The listing builds one solid part. Answer for the finished solid, in the listing's coordinates (mm). Round coordinates to 2 decimals unless told otherwise and drop trailing zeros. Answer in a Markdown table with one row per item. Add a question column.
```python
from build123d import *

# Parameters (mm, degrees)
F1_DEPTH = 3.175
F2_D     = 7.1374
F3_R     = 5.08
F4_D     = 5.6134


# Not quite as in the source:
# - a feature names something its author has since deleted; it is built from what else it names


with BuildPart() as f1:
    # F0 (on Top) → F1 (new body)
    with BuildSketch(Plane.XY):
        Polygon((0, 1181.1), (0, 38.1), (800.1, 38.1), (800.1, 1181.1), (749.3, 1181.1), (749.3, 1155.7), (50.8, 1155.7), (50.8, 1181.1), align=None)
    extrude(amount=F1_DEPTH)

    # F2 (through all)
    with Locations(Plane(origin=(0, 0, 0), x_dir=(1, 0, 0), z_dir=(0, 0, -1))):
        with Locations((25.4, -1168.4), (92.075, -965.2), (117.475, -965.2), (276.225, -965.2), (301.625, -965.2), (460.375, -965.2), (485.775, -965.2), (644.525, -965.2), (669.925, -965.2), (774.7, -1168.4), (669.925, -660.4), (644.525, -660.4), (485.775, -660.4), (460.375, -660.4), (301.625, -660.4), (276.225, -660.4), (117.475, -660.4), (92.075, -660.4), (92.075, -355.6), (117.475, -355.6), (276.225, -355.6), (301.625, -355.6), (460.375, -355.6), (485.775, -355.6), (644.525, -355.6), (669.925, -355.6), (669.925, -50.8), (644.525, -50.8), (485.775, -50.8), (460.375, -50.8), (301.625, -50.8), (276.225, -50.8), (117.475, -50.8), (92.075, -50.8), (774.7, -1079.5), (774.7, -1054.1), (774.7, -774.7), (774.7, -749.3), (774.7, -469.9), (774.7, -444.5), (774.7, -165.1), (774.7, -139.7), (180.975, -965.2), (28.575, -965.2), (212.725, -965.2), (104.775, -1108.075), (288.925, -1108.075), (365.125, -965.2), (396.875, -965.2), (473.075, -1108.075), (549.275, -965.2), (581.025, -965.2), (657.225, -1108.075), (733.425, -965.2), (657.225, -803.275), (473.075, -803.275), (288.925, -803.275), (104.775, -803.275), (28.575, -660.4), (180.975, -660.4), (212.725, -660.4), (365.125, -660.4), (396.875, -660.4), (549.275, -660.4), (581.025, -660.4), (733.425, -660.4), (657.225, -498.475), (473.075, -498.475), (288.925, -498.475), (104.775, -498.475), (28.575, -355.6), (180.975, -355.6), (212.725, -355.6), (365.125, -355.6), (396.875, -355.6), (549.275, -355.6), (581.025, -355.6), (733.425, -355.6), (104.775, -193.675), (288.925, -193.675), (473.075, -193.675), (657.225, -193.675), (733.425, -50.8), (581.025, -50.8), (549.275, -50.8), (396.875, -50.8), (365.125, -50.8), (212.725, -50.8), (180.975, -50.8), (28.575, -50.8)):
            Hole(F2_D / 2)

    # F3
    f3_edges = [f1.edges().sort_by_distance(p)[0] for p in [
        (0, 1181.1, 1.5875),
        (800.1, 1181.1, 1.5875),
        (800.1, 38.1, 1.5875),
        (0, 38.1, 1.5875),
        (50.8, 1181.1, 1.5875),
        (50.8, 1155.7, 1.5875),
        (749.3, 1155.7, 1.5875),
        (749.3, 1181.1, 1.5875),
    ]]
    fillet(f3_edges, radius=F3_R)

    # F4 (through all)
    with Locations(Plane(origin=(0, 0, 0), x_dir=(1, 0, 0), z_dir=(0, 0, -1))):
        with Locations((787.4, -390.525), (787.4, -347.6625), (787.4, -304.8)):
            Hole(F4_D / 2)


solid = f1.part
```
1. Straight lines are drawn through the part: line 1 along Y through (x, z) = (301, 1.6); line 2 along Y through (x, z) = (787.4, 2); line 3 along Y through (x, z) = (272.5, 2.45). For each, find the intervals that lie inside material, in ascending order.
2. This flat-tipped pin is pushed along its axis until it touches: pin 1 (9.5 mm diameter, centred on x = 92.075, y = 50.8, fed in from +Z) (3 decimals). Where does it stop, or does it pass through?
3. The part is cut by section A-A (z = 2). Give the number of separate pieces and of enclosed holes in the cut face, then the cut area to 3 significant figures.
Report:
| question | item | result |
|---|---|---|
| 1 | line 1 | y = 38.1 to 47.29, 54.31 to 352.09, 359.11 to 656.89, 663.91 to 961.69, 968.71 to 1155.7 |
| 1 | line 2 | y = 38.1 to 301.99, 307.61 to 344.86, 350.47 to 387.72, 393.33 to 1181.1 |
| 1 | line 3 | y = 38.1 to 1155.7 |
| 2 | pin 1 | stops at z = 3.175 |
| 3 | separate pieces | 1 |
| 3 | enclosed holes | 93 |
| 3 | area | 893,000 mm^2 |
